```python
from build123d import *

# Parameters (mm, degrees)
SKETCH2_R           = 3.25
BOSS_EXTRUDE1_DEPTH = 13
FILLET1_R           = 3


with BuildPart() as part:
    # Sketch2 → Boss-Extrude1 (new body)
    with BuildSketch(Plane.XY):
        with BuildLine():
            Line((-19.701889993, -1.377690356), (-28.929357458, -2.022937739))
            Line((-28.929357458, -2.022937739), (-28.929357458, 47.977062261))
            Line((-28.929357458, 47.977062261), (28.929357458, 47.977062261))
            Line((28.929357458, 47.977062261), (28.929357458, -2.022937739))
            Line((28.929357458, -2.022937739), (19.701889993, -1.377690356))
            ThreePointArc((19.701889993, -1.377690356), (0, 19.75), (-19.701889993, -1.377690356))
        make_face()
        with Locations(Location((15.209921646, 37.977062261, 0), (0, 0, 180))):
            Circle(SKETCH2_R, mode=Mode.SUBTRACT)
        with Locations(Location((-15.209921646, 37.977062261, 0), (0, 0, 180))):
            Circle(SKETCH2_R, mode=Mode.SUBTRACT)
    extrude(amount=BOSS_EXTRUDE1_DEPTH)

    # Fillet1
    fillet1_edges = [part.edges().sort_by_distance(p)[0] for p in [
        (28.929357458, 22.977062261, 13),
        (-28.929357458, -2.022937739, 6.5),
        (-28.929357458, 47.977062261, 6.5),
        (28.929357458, 47.977062261, 6.5),
        (28.929357458, -2.022937739, 6.5),
        (-28.929357458, 22.977062261, 13),
        (-28.929357458, 22.977062261, 0),
        (28.929357458, 22.977062261, 0),
    ]]
    fillet(fillet1_edges, radius=FILLET1_R)


solid = part.part
```
Could you check a few things on this model? Use its own coordinates, in mm. A direction names the side the tool comes from. Coordinates: 2 decimals unless noted, no trailing zeros. Order: outer loops, then holes, each group sorted by start corner. A loop starts at its lowest first (then second) coordinate and runs counter-clockwise, first axis right, second up. Notation, with made-up numbers: M 8.25,84 L 67.25,84 A27 cw 67.25,112 Z; hole C -26.5,27.25 d6. An arc over 180 degrees is marked long. Use a Markdown table: item, result. Add a question column.
Q1. I want a section at B-B on x = -13. List the corners of the cut face in (y, z) for me, then the cut area to 3 significant figures.
Q2. If I drill on L1, parallel to X at y = 7, z = 8.5; L2, parallel to X at y = 35.5, z = 11.25; L3, parallel to Y at x = -13.5, z = 8.75, over which ranges is the centre line in solid material (lowest first)?
Q3. I want a section at D-D on x = 0. List the corners of the cut face in (y, z) for me, then the cut area to 3 significant figures.
Q4. Which directions (+Z, -Z, +X, -X, +Y, -Y) give clear straight access to the entire face, cutting with the end or side of a thin tool? Please do faces 1 (the cylindrical face through (-14.787, 34.755, 6.409)), 2 (the flat face through (22.75, -1.59, 6.41)).
Q5. We'd pull the mould along X, two halves only. Please class faces 3 (the flat face through (-28.929, 23, 6)), 4 (the cylindrical face through (0.454, 19.745, 6.409)), 5 (the cylindrical face through (28.07, 22.74, 12.1)): pulls with the +X half, pulls with the -X half, needs draft (parallel to the pull), parting line crosses it, or undercut.
Q6. I want a section at A-A on y = 0. List the corners of the cut face in (x, z) for me.
Q7. I'm going to push a flat-ended pin straight in: pin 1 (1 mm diameter, centred on x = 14, z = 11.5, fed in from -Y). Where does the tip first touch, or does it pass through?
Q8. I want a section at C-C on z = 7. List the corners of the cut face in (x, y) for me.
Checked values:
| question | item | result |
|---|---|---|
| 1 | outline | M 14.87,0 L 35.59,0 L 35.59,13 L 14.87,13 Z; M 40.36,0 L 47.98,0 L 47.98,13 L 40.36,13 Z |
| 1 | area | 368 mm² |
| 2 | L1 | -28.93 to -18.47, 18.47 to 28.93 |
| 2 | L2 | -28.66 to -17.31, -13.11 to 13.11, 17.31 to 28.66 |
| 2 | L3 | 14.42 to 35.21, 40.74 to 47.98 |
| 3 | outline | M 19.75,0 L 47.98,0 L 47.98,13 L 19.75,13 Z |
| 3 | area | 367 mm² |
| 4 | face 1 | +Z, -Z |
| 4 | face 2 | +Z, -Z, -Y |
| 5 | face 3 | pulls with the -X half |
| 5 | face 4 | undercut |
| 5 | face 5 | pulls with the +X half |
| 6 | outline | M -28.68,1.81 A3 ccw -25.93,0 L -19.75,0 L -19.75,13 L -25.93,13 A3 ccw -28.68,11.19 Z; M 19.75,0 L 25.93,0 A3 ccw 28.68,1.81 L 28.68,11.19 A3 ccw 25.93,13 L 19.75,13 Z |
| 7 | pin 1 | y = 13.41 |
| 8 | outline | M -28.93,1.19 A3 ccw -25.72,-1.8 L -19.7,-1.38 A19.75 cw long 19.7,-1.38 L 25.72,-1.8 A3 ccw 28.93,1.19 L 28.93,44.98 A3 ccw 25.93,47.98 L -25.93,47.98 A3 ccw -28.93,44.98 Z; hole C -15.21,37.98 d6.5; hole C 15.21,37.98 d6.5 |
